from build123d import *

# Parameters (mm, degrees)
F0_R     = 35
F1_DEPTH = 400
F2_R     = 5
F3_DEPTH = 20
F4_DEPTH = 420
F6_DEPTH = 20
F7_DEPTH = 420


with BuildPart() as f1:
    # F0 (on Front) → F1 (new body)
    with BuildSketch(Plane.XZ):
        Circle(F0_R)
    extrude(amount=F1_DEPTH)

    # F2 (on Front) → F3 (join)
    with BuildSketch(Plane.XZ):
        Circle(F2_R)
    extrude(amount=-F3_DEPTH)

    # F2 (on Front) → F4 (join)
    with BuildSketch(Plane.XZ):
        Circle(F2_R)
    extrude(amount=F4_DEPTH)

    # F5 (on face) → F6 (join, symmetric)
    with BuildSketch(Plane.XZ.offset(400)):
        with BuildLine():
            ThreePointArc((1.3593261446, -4.8116766758), (-0.1474726193, -4.9978247095), (-1.6406738554, -4.723154592))
            Line((-1.6406738554, -4.723154592), (-1.6345586628, -7.9277958721))
            Line((-1.6345586628, -7.9277958721), (1.3655608437, -8.0789448297))
            Line((1.3655608437, -8.0789448297), (1.3593261446, -4.8116766758))
        make_face()
    extrude(amount=F6_DEPTH, both=True)

    # F5 (on face) → F7 (join)
    with BuildSketch(Plane.XZ.offset(400)):
        with BuildLine():
            ThreePointArc((1.3593261446, -4.8116766758), (-0.1474726193, -4.9978247095), (-1.6406738554, -4.723154592))
            Line((-1.6406738554, -4.723154592), (-1.6345586628, -7.9277958721))
            Line((-1.6345586628, -7.9277958721), (1.3655608437, -8.0789448297))
            Line((1.3655608437, -8.0789448297), (1.3593261446, -4.8116766758))
        make_face()
    extrude(amount=-F7_DEPTH)


solid = f1.part
Model file for the job. Use its own axes, mm. A direction names the side the tool comes from. Give positions to 0.01 mm unless a question says otherwise; leave off trailing zeros. Write each loop counter-clockwise with the first axis right and the second up, starting at its lowest first coordinate (ties: lowest second). Pieces come first, ordered by that corner, then holes. Notation, with made-up numbers: M 21,38 L 53,38 A16 ccw 53,55 Z; hole C 73,69 d3. An arc over 180 degrees is marked long. One line per item, written item: value. Start each with the question number.
Q1. Saw through at A-A, the plane z = 0. Write the cut outline in (x, y), plus the area to 3 significant figures.
Q2. Saw through at D-D, the plane z = 19. Write the cut outline in (x, y).
Q3. Drop flat-ended pins along their axis: pin 1 Ø12 at (x, y) = (11, -267.5) entering from +Z; pin 2 Ø10 at (y, z) = (-107.5, -10) entering from -X; pin 3 Ø6 at (y, z) = (-157, 18) entering from -X. Give the stop position or say it passes through.
Q4. 3-axis set-ups, long thin cutter, end or side, ignore diameter. For faces 1 (the cylindrical face through (0, 10, 5)), 2 (the cylindrical face through (0, -410, 5)), 3 (the flat face through (0, -420, 0)): which of +Z, -Z, +X, -X, +Y, -Y reach the whole face in a straight line?
Q5. Saw through at C-C, the plane x = 19.5. Write the cut outline in (y, z).
Q6. Saw through at B-B, the plane y = -100.5. Write the cut outline in (x, z).
Q7. Probe probe 1 along Y at (x, z) = (30.5, -13); probe 2 along X at (y, z) = (-69, 1); probe 3 along Z at (x, y) = (23, -69.5). List the from-to ranges inside material, lowest first. Write a range as [from, to].
Output values:
1. outline: M -35,-400 L -5,-400 L -5,-420 L 5,-420 L 5,-400 L 35,-400 L 35,0 L 5,0 L 5,20 L -5,20 L -5,0 L -35,0 Z
1. area: 28,400 mm²
2. outline: M -29.39,-400 L 29.39,-400 L 29.39,0 L -29.39,0 Z
3. pin 1: stops at z = 34.64
3. pin 2: stops at x = -34.64
3. pin 3: stops at x = -31.62
4. face 1: +Y
4. face 2: -Y
4. face 3: +Z, -Z, +X, -X, -Y
5. outline: M -400,-29.06 L 0,-29.06 L 0,29.06 L -400,29.06 Z
6. outline: C 0,0 d70
7. probe 1: y = [-400, 0]
7. probe 2: x = [-34.99, 34.99]
7. probe 3: z = [-26.38, 26.38]
